Model file for the job. Use its own axes, mm. Give positions to 0.01 mm unless a question says otherwise; leave off trailing zeros. Order: outer loops, then holes, each group sorted by start corner. A loop starts at its lowest first (then second) coordinate and runs counter-clockwise, first axis right, second up. Notation, with made-up numbers: (6.5, 15) -> (54.5, 15) arc R19 ccw to (54.5, 48) -> close; hole circle Ø9 at (40.5, 42.25). An arc over 180 degrees is marked (long way). Answer in a Markdown table with one row per item. Add a question column.
Autodesk Inventor part; units mm, degrees
ref_plane "YZ Plane" through (0, 0, 0) normal (1, 0, 0) x (0, 1, 0)
ref_plane "XZ Plane" through (0, 0, 0) normal (0, 1, 0) x (-1, 0, 0)
ref_plane "XY Plane" through (0, 0, 0) normal (0, 0, 1) x (1, 0, 0)
sketch "Эскиз1" plane through (0, 0, 0) normal (0, 0, 1) x (1, 0, 0)
  line L0 (10, -17.5) -> (-10, -17.5)
  line L1 (-10, -17.5) -> (-10, 17.5)
  line L2 (-10, 17.5) -> (10, 17.5)
  line L3 (10, 17.5) -> (10, -17.5)
  line L4 (10, -17.5) -> (-10, 17.5) construction
  line L5 (-10, -17.5) -> (10, 17.5) construction
  point P0 (0, 0)
  dimension "d0" = 20
  dimension "d1" = 35
extrude "Выдавливание1" add sketch "Эскиз1" along normal blind 2
fillet "Сопряжение1" radius 2 4 edges at (-10, 17.5, 1) (10, 17.5, 1) (10, -17.5, 1) (-10, -17.5, 1)
sketch "Эскиз2" plane through (0, 0, 0) normal (0, 0, -1) x (-1, 0, 0)
  circle A0 centre (-7, 7.5) radius 2.1
  circle A1 centre (-7, -14.5) radius 2.1
  line L0 (-5.7982, 10.5) -> (-5.7982, 18.5)
  line L1 (-5.7982, 18.5) -> (-8, 18.5)
  arc A2 (-8, 18.5) -> (-11, 15.5) centre (-8, 15.5) ccw
  line L2 (-11, 15.5) -> (-11, 2.5)
  arc A3 (-11, -15.5) -> (-8, -18.5) centre (-8, -15.5) ccw
  line L3 (-8, -18.5) -> (8, -18.5)
  arc A4 (8, -18.5) -> (11, -15.5) centre (8, -15.5) ccw
  line L4 (11, 6) -> (11, 10.5)
  line L5 (11, 10.5) -> (-5.7982, 10.5)
  circle A5 centre (-7, -14.5) radius 1.6
  circle A6 centre (-7, 7.5) radius 1.6
  line L6 (-11, 2.5) -> (-4, 2.5)
  line L7 (-4, 2.5) -> (-4, -9.5)
  line L8 (-4, -9.5) -> (-11, -9.5)
  line L9 (11, -6) -> (4, -6)
  line L10 (4, -6) -> (4, 6)
  line L11 (4, 6) -> (11, 6)
  line L12 (-11, -9.5) -> (-11, -15.5)
  line L13 (11, -15.5) -> (11, -6)
  point P0 (0, 0)
  dimension "d5" = 3.2
  dimension "d6" = 3.2
extrude "Выдавливание2" cut sketch "Эскиз2" against normal blind 2 contours A5 | A6
properties part number "comutation_motorboard"
Item 1: Saw through at C-C on z = 1.3. List the corners of the cut face in (x, y), plus the area to 3 significant figures.
Item 2: Pin check, flat tip, straight feed: pin 1 Ø3.5 at (x, y) = (7, 7.5) entering from -Z. Stop position of the tip, or through.
Item 3: Two-plate mould, pull along Y, no slides. Class faces 1 (the flat face through (0, 0, 0)), 2 (the flat face through (0, 17.5, 1)), 3 (the cylindrical face through (7.35, 5.94, 0.99)): pulls with the +Y half, pulls with the -Y half, needs draft (parallel to the pull), parting line crosses it, or undercut.
Item 4: Wall check: line 1 (Y direction, x = 7, z = 1.2); line 2 (Y direction, x = 9, z = 1.45); line 3 (X direction, y = 16, z = 1.2). Give the ranges that are in metal, low to high.
Item 5: Saw through at A-A on y = -14.5. List the corners of the cut face in (x, z).
Item 6: Saw through at B-B on x = 7. List the corners of the cut face in (y, z).
Evaluation:
| question | item | result |
|---|---|---|
| 1 | outline | (-10, -15.5) arc R2 ccw to (-8, -17.5) -> (8, -17.5) arc R2 ccw to (10, -15.5) -> (10, 15.5) arc R2 ccw to (8, 17.5) -> (-8, 17.5) arc R2 ccw to (-10, 15.5) -> close; hole circle Ø3.2 at (7, -14.5); hole circle Ø3.2 at (7, 7.5) |
| 1 | area | 680 mm2 |
| 2 | pin 1 | stops at z = 0 |
| 3 | face 1 | needs draft |
| 3 | face 2 | pulls with the +Y half |
| 3 | face 3 | undercut |
| 4 | line 1 | y = -17.5 to -16.1, -12.9 to 5.9, 9.1 to 17.5 |
| 4 | line 2 | y = -17.23 to 17.23 |
| 4 | line 3 | x = -9.94 to 9.94 |
| 5 | outline | (-10, 0) -> (5.4, 0) -> (5.4, 2) -> (-10, 2) -> close; (8.6, 0) -> (10, 0) -> (10, 2) -> (8.6, 2) -> close |
| 6 | outline | (-17.5, 0) -> (-16.1, 0) -> (-16.1, 2) -> (-17.5, 2) -> close; (-12.9, 0) -> (5.9, 0) -> (5.9, 2) -> (-12.9, 2) -> close; (9.1, 0) -> (17.5, 0) -> (17.5, 2) -> (9.1, 2) -> close |
